Can you work these out from the drawing? Everything is in mm from the part's minimum corner. Give positions to 0.01 mm unless a question says otherwise; leave off trailing zeros. Write each loop counter-clockwise with the first axis right and the second up, starting at its lowest first coordinate (ties: lowest second). Pieces come first, ordered by that corner, then holes. Notation, with made-up numbers: (7, 72) - (12, 72) arc R14 cw to (12, 80) - close; hole circle Ø11 at (69.25, -26). An arc over 180 degrees is marked (long way). Use a Markdown table: item, result.
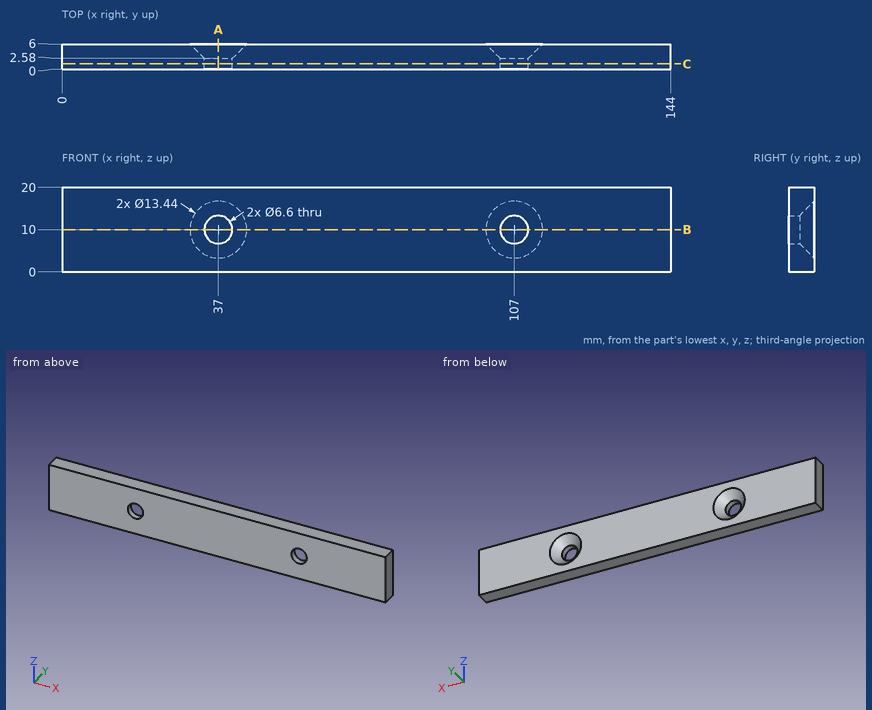
Item 1: I need wall thicknesses on line 1 along X through (y, z) = (0.7, 10); line 2 along Z through (x, y) = (37, 1.3); line 3 along X through (y, z) = (4.05, 9.5). Which ranges of each line are inside material? Lowest first, please. Write a range as [from, to].
Values:
| item | result |
|---|---|
| line 1 | x = [0, 33.7], [40.3, 103.7], [110.3, 144] |
| line 2 | z = [0, 6.7], [13.3, 20] |
| line 3 | x = [0, 32.26], [41.74, 102.26], [111.74, 144] |
Item 2: If we section it at A-A, the plane x = 37: Write out the boundary of the cut face in (y, z), plus the area to 3 significant figures.
Values:
| item | result |
|---|---|
| outline | (0, 0) - (6, 0) - (6, 3.28) - (2.58, 6.7) - (0, 6.7) - close; (0, 13.3) - (2.58, 13.3) - (6, 16.72) - (6, 20) - (0, 20) - close |
| area | 68.7 mm2 |
Item 3: If we section it at B-B, the plane z = 10: Write out the boundary of the cut face in (x, y), plus the area to 3 significant figures.
Values:
| item | result |
|---|---|
| outline | (0, 0) - (33.7, 0) - (33.7, 2.58) - (30.28, 6) - (0, 6) - close; (40.3, 0) - (103.7, 0) - (103.7, 2.58) - (100.28, 6) - (43.72, 6) - (40.3, 2.58) - close; (110.3, 0) - (144, 0) - (144, 6) - (113.72, 6) - (110.3, 2.58) - close |
| area | 761 mm2 |
Item 4: If we section it at C-C, the plane y = 1.3: Write out the boundary of the cut face in (x, z).
Values:
| item | result |
|---|---|
| outline | (0, 0) - (144, 0) - (144, 20) - (0, 20) - close; hole circle Ø6.6 at (37, 10); hole circle Ø6.6 at (107, 10) |
Item 5: Will this pin go through, and if not, where does the flat tip stop? pin 1 Ø4 at (x, z) = (37, 10) entering from +Y.
Values:
| item | result |
|---|---|
| pin 1 | passes through |
